Geometry: final body of the model. Coordinates: model frame, mm. Face numbers are marked on the shaded views. A direction names the side the tool comes from. Coordinates: 2 decimals unless noted, no trailing zeros. Write each loop counter-clockwise with the first axis right and the second up, starting at its lowest first coordinate (ties: lowest second). Pieces come first, ordered by that corner, then holes.
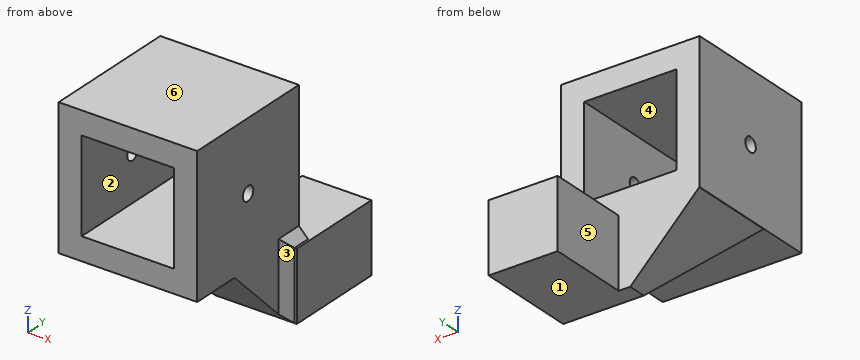
from build123d import *

# Parameters (mm, degrees)
SKETCH4_W                = 20.1
SKETCH4_H                = 20.1
BOSS_EXTRUDE6_DEPTH      = 5
BOSS_EXTRUDE7_DEPTH      = 15
BOSS_EXTRUDE7_DEPTH_BACK = 15
SKETCH4_4_W              = 30.1
SKETCH4_4_H              = 30.1
SKETCH4_4_W_2            = 20.1
SKETCH4_4_H_2            = 20.1
SKETCH5_R                = 1.55
CUT_EXTRUDE1_DEPTH       = 54
BOSS_EXTRUDE8_START      = 15
SKETCH4_5_W              = 15
SKETCH4_5_H              = 15
BOSS_EXTRUDE8_DEPTH      = 18
SKETCH6_W                = 17.5
SKETCH6_H                = 15
BOSS_EXTRUDE9_DEPTH      = 4
CHAMFER1_SIZE            = 15
CHAMFER2_SIZE            = 15
CHAMFER3_SIZE            = 2


with BuildPart() as part:
    # Sketch4 → Boss-Extrude6 (new body)
    with BuildSketch(Plane(origin=(0, 310, 0), x_dir=(1, 0, 0), z_dir=(0, 1, 0))):
        Polygon((5, 25.1), (-7.5, 25.1), (-25.1, 25.1), (-25.1, -5), (5, -5), align=None)
        with Locations((-10.05, 10.05)):
            Rectangle(SKETCH4_W, SKETCH4_H, mode=Mode.SUBTRACT)
    extrude(amount=-BOSS_EXTRUDE6_DEPTH)

    # Sketch4<4> → Boss-Extrude7 (add, two sides: drawn at the far end of the back side and taken through both)
    with BuildSketch(Plane(origin=(0, 310, 0), x_dir=(1, 0, 0), z_dir=(0, 1, 0)).offset(-BOSS_EXTRUDE7_DEPTH_BACK)):
        with Locations((-10.05, 10.05)):
            Rectangle(SKETCH4_4_W, SKETCH4_4_H)
        with Locations((-10.05, 10.05)):
            Rectangle(SKETCH4_4_W_2, SKETCH4_4_H_2, mode=Mode.SUBTRACT)
    extrude(amount=BOSS_EXTRUDE7_DEPTH + BOSS_EXTRUDE7_DEPTH_BACK)

    # Sketch5 → Cut-Extrude1 (cut)
    with BuildSketch(Plane(origin=(5, 0, 0), x_dir=(0, 0, -1), z_dir=(1, 0, 0))):
        with Locations(Location((10.05, 310, 0), (0, 0, 180))):
            Circle(SKETCH5_R)
    extrude(amount=-CUT_EXTRUDE1_DEPTH, mode=Mode.SUBTRACT)



with BuildPart() as body_2:
    # Sketch4<5> → Boss-Extrude8 (new body)
    with BuildSketch(Plane(origin=(0, 310, 0), x_dir=(1, 0, 0), z_dir=(0, 1, 0)).offset(BOSS_EXTRUDE8_START)):
        with Locations((0, 32.6)):
            Rectangle(SKETCH4_5_W, SKETCH4_5_H)
    extrude(amount=BOSS_EXTRUDE8_DEPTH)


with BuildPart() as part_1:
    add(part.part)

    add(body_2.part)  # Boss-Extrude9 merges body 2
    # Sketch6 → Boss-Extrude9 (add)
    with BuildSketch(Plane(origin=(0, 325, 0), x_dir=(1, 0, 0), z_dir=(0, 1, 0))):
        with Locations((-1.25, 32.6)):
            Rectangle(SKETCH6_W, SKETCH6_H)
    extrude(amount=-BOSS_EXTRUDE9_DEPTH)

    # Chamfer1
    chamfer1_edges = [part_1.edges().sort_by_distance(p)[0] for p in [
        (-2.5, 321, -25.1),
    ]]
    chamfer(chamfer1_edges, length=CHAMFER1_SIZE - 0.0001)  # a hair under: the kernel refuses the full size

    # Chamfer2
    chamfer2_edges = [part_1.edges().sort_by_distance(p)[0] for p in [
        (-10, 315.50005, -25.1),
    ]]
    chamfer(chamfer2_edges, length=CHAMFER2_SIZE - 0.0001)  # a hair under: the kernel refuses the full size

    # Chamfer3
    chamfer3_edges = [part_1.edges().sort_by_distance(p)[0] for p in [
        (5, 321, -32.59995),
        (5, 323, -25.1),
    ]]
    chamfer(chamfer3_edges, length=CHAMFER3_SIZE)


solid = part_1.part
Item 1: Material intervals for probe 1 along Y at (x, z) = (-22.85, -10.05); probe 2 along Z at (x, y) = (-13.5, 298), sorted ascending.
Derived:
probe 1: y = 295 to 308.45, 311.55 to 325
probe 2: z = -25.1 to -20.1, 0 to 5
Item 2: Set-up query: the marked faces 4, 5 and 6. Return all of +Z, -Z, +X, -X, +Y, -Y with unobstructed straight access to the full face (end or side cutting, diameter ignored); none if empty.
Derived:
face 4: +Y, -Y
face 5: +Z, -Z, -X, +Y
face 6: +Z, +X, -X, +Y, -Y
Item 3: Section A-A, the plane z = -1.5. Output: boundary loops of the cut face in (x, y).
Derived:
outline: (-25.1, 295) - (-20.1, 295) - (-20.1, 325) - (-25.1, 325) - close; (0, 295) - (5, 295) - (5, 325) - (0, 325) - close
Item 4: Pin query (flat end, axial travel): pin 1 (10 mm diameter, centred on x = -9.5, z = -20, fed in from -Y); pin 2 (8 mm diameter, centred on x = -20.5, z = -0.5, fed in from +Y); pin 3 (7.5 mm diameter, centred on y = 335, z = -34, fed in from -X); pin 4 (9 mm diameter, centred on x = -9, y = 312.5, fed in from -Z). Return the tip coordinate at first contact, or that it passes through.
Derived:
pin 1: stops at y = 295
pin 2: stops at y = 325
pin 3: stops at x = -7.5
pin 4: stops at z = -36.1
Item 5: Pull-direction query (X, two-part tool) for the marked faces 1, 2 and 3; classes: released by +X, released by -X, zero draft, split by the parting line, or undercut.
Derived:
face 1: zero draft
face 2: undercut
face 3: released by +X
Item 6: Section D-D, the plane z = -10.05. Output: boundary loops of the cut face in (x, y), plus the area to 3 significant figures.
Derived:
outline: (-25.1, 295) - (-20.1, 295) - (-20.1, 308.45) - (-25.1, 308.45) - close; (-25.1, 311.55) - (-20.1, 311.55) - (-20.1, 325) - (-25.1, 325) - close; (0, 295) - (5, 295) - (5, 308.45) - (0, 308.45) - close; (0, 311.55) - (5, 311.55) - (5, 325) - (0, 325) - close
area: 269 mm2
